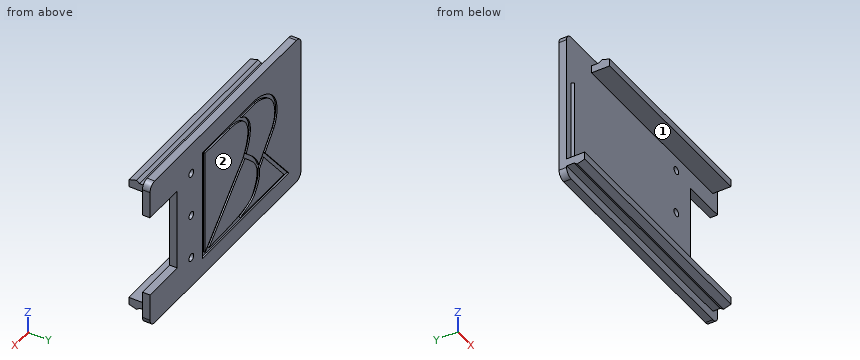
```python
from build123d import *

# Parameters (mm, degrees)
BOSS_EXTRUDE1_DEPTH             = 1
BOSS_EXTRUDE2_DEPTH             = 2.4
BOSS_EXTRUDE3_REACH             = 18.1
BOSS_EXTRUDE3_DIRECTION_2_REACH = 18.1
BOSS_EXTRUDE4_DEPTH             = 5.3
FILLET1_R                       = 1
SKETCH5_W                       = 1
SKETCH5_H                       = 2.4
BOSS_EXTRUDE5_DEPTH             = 0.8
CUT_EXTRUDE1_DEPTH              = 0.2
BOSS_EXTRUDE6_DEPTH             = 11.5
SKETCH12_R                      = 0.5
CUT_EXTRUDE6_DEPTH              = 4.4


with BuildPart() as part:
    # Sketch1 → Boss-Extrude1 (new body)
    with BuildSketch(Plane(origin=(0, 0, 0), x_dir=(1, 0, 0), z_dir=(0, 1, 0))):
        Polygon((16.1, 5.5), (10.3, 5.5), (10.3, -5.5), (16.1, -5.5), (16.1, -10.1), (-16.1, -10.1), (-16.1, 10.1), (16.1, 10.1), align=None)
    extrude(amount=BOSS_EXTRUDE1_DEPTH)

    # Sketch2 → Boss-Extrude2 (add)
    with BuildSketch(Plane.XZ):
        Polygon((15.1, 8.9), (-10.8, 8.9), (-10.8, 7.9), (14.1, 7.9), (15.1, 7.9), align=None)
        Polygon((15.1, -8.9), (-15.3, -8.9), (-15.3, -7.9), (-14.3, -7.9), (14.1, -7.9), (15.1, -7.9), align=None)
    extrude(amount=BOSS_EXTRUDE2_DEPTH)

    # Boss-Extrude3: up to this face of the body (flat: up to its plane)
    boss_extrude3_end = Plane(part.part.faces().sort_by_distance((-10.8, -1.2, 8.4))[0])
    # Sketch3 → Boss-Extrude3 (add, up to the picked face)
    with BuildSketch(Plane(origin=(0, 0, 0), x_dir=(0, 0, -1), z_dir=(1, 0, 0)), mode=Mode.PRIVATE) as boss_extrude3_sk1:
        Polygon((8.9, -2.4), (9.2, -1.4), (8.9, -1), align=None)
    boss_extrude3_tool1 = split(extrude(boss_extrude3_sk1.sketch, amount=-BOSS_EXTRUDE3_REACH, mode=Mode.PRIVATE), bisect_by=boss_extrude3_end, keep=Keep.BOTH, mode=Mode.PRIVATE)
    add(boss_extrude3_tool1.solids().sort_by_distance((0, -1.6, -9))[0])
    # Sketch3 → Boss-Extrude3 (add, up to the picked face)
    with BuildSketch(Plane(origin=(0, 0, 0), x_dir=(0, 0, -1), z_dir=(1, 0, 0)), mode=Mode.PRIVATE) as boss_extrude3_sk2:
        Polygon((-8.9, -1), (-8.9, -2.4), (-9.2, -1.4), align=None)
    boss_extrude3_tool2 = split(extrude(boss_extrude3_sk2.sketch, amount=-BOSS_EXTRUDE3_REACH, mode=Mode.PRIVATE), bisect_by=boss_extrude3_end, keep=Keep.BOTH, mode=Mode.PRIVATE)
    add(boss_extrude3_tool2.solids().sort_by_distance((0, -1.6, 9))[0])

    # Boss-Extrude3 direction 2: up to this face of the body (flat: up to its plane)
    boss_extrude3_direction_2_end = Plane(part.part.faces().sort_by_distance((15.1, -1.2, -8.4))[0])
    # Sketch3 → Boss-Extrude3 direction 2 (add, up to the picked face)
    with BuildSketch(Plane(origin=(0, 0, 0), x_dir=(0, 0, -1), z_dir=(1, 0, 0)), mode=Mode.PRIVATE) as boss_extrude3_direction_2_sk1:
        Polygon((8.9, -2.4), (9.2, -1.4), (8.9, -1), align=None)
    boss_extrude3_direction_2_tool1 = split(extrude(boss_extrude3_direction_2_sk1.sketch, amount=BOSS_EXTRUDE3_DIRECTION_2_REACH, mode=Mode.PRIVATE), bisect_by=boss_extrude3_direction_2_end, keep=Keep.BOTH, mode=Mode.PRIVATE)
    add(boss_extrude3_direction_2_tool1.solids().sort_by_distance((0, -1.6, -9))[0])
    # Sketch3 → Boss-Extrude3 direction 2 (add, up to the picked face)
    with BuildSketch(Plane(origin=(0, 0, 0), x_dir=(0, 0, -1), z_dir=(1, 0, 0)), mode=Mode.PRIVATE) as boss_extrude3_direction_2_sk2:
        Polygon((-8.9, -1), (-8.9, -2.4), (-9.2, -1.4), align=None)
    boss_extrude3_direction_2_tool2 = split(extrude(boss_extrude3_direction_2_sk2.sketch, amount=BOSS_EXTRUDE3_DIRECTION_2_REACH, mode=Mode.PRIVATE), bisect_by=boss_extrude3_direction_2_end, keep=Keep.BOTH, mode=Mode.PRIVATE)
    add(boss_extrude3_direction_2_tool2.solids().sort_by_distance((0, -1.6, 9))[0])

    # Sketch4 → Boss-Extrude4 (add)
    with BuildSketch(Plane.ZY.offset(10.8)):
        Polygon((-8.9, -2.4), (-8.9, -1), (-9.2, -1.4), align=None)
    extrude(amount=BOSS_EXTRUDE4_DEPTH)

    # Fillet1
    fillet1_edges = [part.edges().sort_by_distance(p)[0] for p in [
        (-16.1, 0.5, 10.1),
        (16.1, 0.5, 10.1),
        (16.1, 0.5, -10.1),
        (-16.1, 0.5, -10.1),
    ]]
    fillet(fillet1_edges, radius=FILLET1_R)

    # Sketch5 → Boss-Extrude5 (add)
    with BuildSketch(Plane.ZY.offset(15.3)):
        with Locations((-8.4, -1.2)):
            Rectangle(SKETCH5_W, SKETCH5_H)
    extrude(amount=BOSS_EXTRUDE5_DEPTH)

    # Sketch9 → Cut-Extrude1 (cut)
    with BuildSketch(Plane(origin=(0, 1, 0), x_dir=(1, 0, 0), z_dir=(0, 1, 0))):
        with BuildLine():
            add(Edge.make_bspline(
                [(-3.342815403, -6.898771532), (-3.392032296, -6.876638055), (-3.827458148, -6.670816542), (-4.519691405, -6.171060382), (-5.129218139, -5.217739053), (-5.348913685, -4.118130523), (-5.230008041, -2.951908877), (-4.894461229, -1.967151288), (-4.588355912, -1.345070717), (-4.453256479, -1.098754494), (-4.417927521, -1.036087622), (-4.4033747, -1.01056214)],
                knots=[0.234294725, 0.234294725, 0.234294725, 0.234294725, 0.249919787, 0.375, 0.5, 0.625, 0.75, 0.875, 0.931300557, 0.942750464, 0.95062349, 0.95062349, 0.95062349, 0.95062349], degree=3))
            add(Edge.make_bspline(
                [(-3.342815403, -6.898771532), (-2.542251184, -7.287796887), (-1.658619274, -7.383876714)],
                knots=[0, 0, 0, 1, 1, 1], degree=2))
            Line((-1.658619274, -7.383876714), (-0.948898515, -7.383876714))
            Line((-0.948898515, -7.383876714), (4.858590941, -7.383876714))
            Line((4.858590941, -7.383876714), (4.858590941, 7.737734352))
            Line((4.858590941, 7.737734352), (-3.156218351, 7.262620046))
            add(Edge.make_bspline(
                [(-3.156218351, 7.262620046), (-4.204686525, 6.965216897), (-5.726735189, 6.631756812), (-7.011707154, 4.951403609), (-7.402848959, 3.939339374), (-7.264734741, 2.979074857)],
                knots=[0.007330404, 0.007330404, 0.007330404, 0.007330404, 0.225500981, 0.280065017, 0.552970764, 0.552970764, 0.552970764, 0.552970764], degree=3))
            Line((-7.264734741, 2.979074857), (-7.117659595, 2.367238768))
            add(Edge.make_bspline(
                [(-7.117659595, 2.367238768), (-6.960941749, 1.890945903), (-6.272373332, 0.577066844), (-5.102929425, -0.364874806), (-4.4033747, -1.01056214)],
                knots=[0.609519995, 0.609519995, 0.609519995, 0.609519995, 0.739586039, 0.961717779, 0.961717779, 0.961717779, 0.961717779], degree=3))
        make_face()
        with BuildLine():
            Line((-3.689882661, -0.799866909), (4.352426166, 7.237734352))
            Line((4.352426166, 7.237734352), (4.352426166, -6.898771532))
            Line((4.352426166, -6.898771532), (0.040224346, -6.898771532))
            Line((0.040224346, -6.898771532), (-0.948898515, -6.898771532))
            add(Edge.make_bspline(
                [(-0.948898515, -6.898771532), (-5.034514831, -6.847494081), (-5.677385917, -3.860270153), (-3.689882661, -0.799866909)],
                knots=[0, 0, 0, 0, 1, 1, 1, 1], degree=3))
        make_face(mode=Mode.SUBTRACT)
        with BuildLine():
            Line((3.506059361, 7.097194921), (-4.128123279, -0.530951144))
            add(Edge.make_bspline(
                [(3.506059361, 7.097194921), (-3.269089821, 7.048794638), (-5.221862409, 6.449276012), (-6.471825808, 4.765768499), (-7.041574265, 2.901212273), (-5.99383179, 1.096583313), (-4.827678003, 0.11473619), (-4.128123279, -0.530951144)],
                knots=[0.007330404, 0.007330404, 0.007330404, 0.007330404, 0.225500981, 0.28162106, 0.568531193, 0.739586039, 0.961717779, 0.961717779, 0.961717779, 0.961717779], degree=3))
        make_face(mode=Mode.SUBTRACT)
        with BuildLine():
            add(Edge.make_bspline(
                [(-3.342815403, -6.898771532), (-2.542251184, -7.287796887), (-1.658619274, -7.383876714)],
                knots=[0, 0, 0, 1, 1, 1], degree=2))
            Line((-3.342815403, -6.898771532), (-6.38229421, -6.898771532))
            add(Edge.make_bspline(
                [(-9.901940455, -1.035163603), (-10.745351374, -2.262822828), (-10.813877235, -5.298026757), (-7.511264228, -6.800208927), (-6.38229421, -6.898771532)],
                knots=[0, 0, 0, 0, 0.624222909, 1, 1, 1, 1], degree=3))
            Line((-9.901940455, -1.035163603), (-7.799125954, 1.534484145))
            Line((-7.799125954, 1.534484145), (-7.117659595, 2.367238768))
            Line((-7.117659595, 2.367238768), (-7.264734741, 2.979074857))
            Line((-7.264734741, 2.979074857), (-8.121685172, 1.931877995))
            Line((-8.121685172, 1.931877995), (-12.428377088, 7.237734352))
            Line((-12.428377088, 7.237734352), (-3.156218351, 7.262620046))
            Line((-3.156218351, 7.262620046), (4.858590941, 7.737734352))
            Line((4.858590941, 7.737734352), (-13.478199155, 7.737734352))
            Line((-13.478199155, 7.737734352), (-8.434565478, 1.523963693))
            Line((-8.434565478, 1.523963693), (-10.290254207, -0.743695372))
            add(Edge.make_bspline(
                [(-10.290254207, -0.743695372), (-10.681696867, -1.313474801), (-11.163382472, -2.664450315), (-10.847207421, -4.528853246), (-9.910083857, -5.835484729), (-8.881232555, -6.617480767), (-7.669601654, -7.167356574), (-6.83032417, -7.346607487), (-6.403429612, -7.383876714)],
                knots=[-0.002843331, -0.002843331, -0.002843331, -0.002843331, 0.248451523, 0.499746376, 0.625393803, 0.75104123, 0.876688657, 1.002336083, 1.002336083, 1.002336083, 1.002336083], degree=3))
            Line((-6.403429612, -7.383876714), (-1.658619274, -7.383876714))
        make_face()
    extrude(amount=-CUT_EXTRUDE1_DEPTH, mode=Mode.SUBTRACT)

    # Sketch11 → Boss-Extrude6 (add)
    with BuildSketch(Plane.XY.offset(-7.9)):
        Polygon((-15.1, 0), (-14.6, 0), (-14.85, -0.3), align=None)
    extrude(amount=BOSS_EXTRUDE6_DEPTH)

    # Sketch12 → Cut-Extrude6 (cut, through all)
    with BuildSketch(Plane(origin=(0, 1, 0), x_dir=(1, 0, 0), z_dir=(0, 1, 0))):
        with Locations((7.3, 0)):
            Circle(SKETCH12_R)
        with Locations((7.3, -6)):
            Circle(SKETCH12_R)
        with Locations((7.3, 6)):
            Circle(SKETCH12_R)
    extrude(amount=-CUT_EXTRUDE6_DEPTH, mode=Mode.SUBTRACT)


solid = part.part
```
The listing builds one solid part. Answer for the finished solid, in the listing's coordinates (mm). Face numbers are marked on the shaded views. Give positions to 0.01 mm unless a question says otherwise; leave off trailing zeros. Order: outer loops, then holes, each group sorted by start corner. A loop starts at its lowest first (then second) coordinate and runs counter-clockwise, first axis right, second up.
1) Determine the mould class of the marked faces 1 and 2 for opening direction Z: pulls with the +Z half, pulls with the -Z half, needs draft (parallel to the pull), parting line crosses it, or undercut.
Reported:
face 1: undercut
face 2: needs draft
2) Find section B-B on x = 7.3. Write down the section's boundary in (y, z), then the cut area to 3 significant figures.
Reported:
outline: (-2.4, -8.9) - (-1.4, -9.2) - (-1, -8.9) - (0, -8.9) - (0, -10.1) - (1, -10.1) - (1, -6.5) - (0, -6.5) - (0, -7.9) - (-2.4, -7.9) - close; (-2.4, 7.9) - (0, 7.9) - (0, 6.5) - (1, 6.5) - (1, 10.1) - (0, 10.1) - (0, 8.9) - (-1, 8.9) - (-1.4, 9.2) - (-2.4, 8.9) - close; (0, -5.5) - (1, -5.5) - (1, -0.5) - (0, -0.5) - close; (0, 0.5) - (1, 0.5) - (1, 5.5) - (0, 5.5) - close
area: 22.4 mm2
3) Given P1, Ø1.2, axis at x = -3.5, y = -1, coming from the +Z side; P2, Ø1.5, axis at y = -0.5, z = -0.5, coming from the +X side; P3, Ø0.7, axis at y = -0.5, z = 8.5, coming from the -X side, each flat-ended and moving along its own axis, determine where each tip first touches the part or whether it passes through.
Reported:
P1: stops at z = 9.2
P2: stops at x = 10.3
P3: stops at x = -10.8
4) Find section A-A on x = 13. Write down the section's boundary in (y, z).
Reported:
outline: (-2.4, -8.9) - (-1.4, -9.2) - (-1, -8.9) - (0, -8.9) - (0, -10.1) - (1, -10.1) - (1, -5.5) - (0, -5.5) - (0, -7.9) - (-2.4, -7.9) - close; (-2.4, 7.9) - (0, 7.9) - (0, 5.5) - (1, 5.5) - (1, 10.1) - (0, 10.1) - (0, 8.9) - (-1, 8.9) - (-1.4, 9.2) - (-2.4, 8.9) - close
5) Consider line 1 along Z through (x, y) = (7.3, 0.75); line 2 along X through (y, z) = (0.4, -6); line 3 along X through (y, z) = (0.55, 0). Determine where each line is inside the solid, lowest interval first.
Reported:
line 1: z = -10.1 to -6.5, -5.5 to -0.5, 0.5 to 5.5, 6.5 to 10.1
line 2: x = -16.1 to 6.8, 7.8 to 16.1
line 3: x = -16.1 to 6.8, 7.8 to 10.3
6) Find section C-C on z = -8.5. Write down the section's boundary in (x, y).
Reported:
outline: (-16.1, -2.4) - (15.1, -2.4) - (15.1, 0) - (16.1, 0) - (16.1, 1) - (-16.1, 1) - close
7) Find section D-D on x = -12. Write down the section's boundary in (y, z), then the cut area to 3 significant figures.
Reported:
outline: (-2.4, -8.9) - (-1.4, -9.2) - (-1, -8.9) - (0, -8.9) - (0, -10.1) - (1, -10.1) - (1, -7.74) - (0.8, -7.74) - (0.8, -7.24) - (1, -7.24) - (1, -6.71) - (0.8, -6.71) - (0.8, -5.92) - (1, -5.92) - (1, 10.1) - (0, 10.1) - (0, -7.9) - (-2.4, -7.9) - close
area: 22.6 mm2
